```python
from build123d import *

# Parameters (mm, degrees)
F1_DEPTH = 561.975
F2_R     = 2.6162
F3_DEPTH = 25.4


with BuildPart() as f1:
    # F0 (on Right) → F1 (new body)
    with BuildSketch(Plane.YZ):
        with BuildLine():
            Line((0, -19.05), (0, -3.175))
            ThreePointArc((0, -3.175), (-0.929936, -0.929936), (-3.175, 0))
            Line((-3.175, 0), (-3.175, -25.4))
            Line((-3.175, -25.4), (22.225, -25.4))
            ThreePointArc((22.225, -25.4), (21.295064, -23.154936), (19.05, -22.225))
            Line((19.05, -22.225), (3.175, -22.225))
            ThreePointArc((3.175, -22.225), (0.929936, -21.295064), (0, -19.05))
        make_face()
    extrude(amount=-F1_DEPTH)

    # F2 (on face) → F3 (cut)
    with BuildSketch(Plane(origin=(0, 0, 0), x_dir=(-1, 0, 0), z_dir=(0, 1, 0))):
        with Locations((10.31875, -11.1125)):
            Circle(F2_R)
        with Locations((280.9875, -11.1125)):
            Circle(F2_R)
        with Locations((551.65625, -11.1125)):
            Circle(F2_R)
        with Locations((128.5875, -11.1125)):
            Circle(F2_R)
        with Locations((204.7875, -11.1125)):
            Circle(F2_R)
        with Locations((357.1875, -11.1125)):
            Circle(F2_R)
        with Locations((433.3875, -11.1125)):
            Circle(F2_R)
        with Locations((509.5875, -11.1125)):
            Circle(F2_R)
        with Locations((52.3875, -11.1125)):
            Circle(F2_R)
        with Locations((33.3375, -11.1125)):
            Circle(F2_R)
        with Locations((71.4375, -11.1125)):
            Circle(F2_R)
        with Locations((490.5375, -11.1125)):
            Circle(F2_R)
        with Locations((528.6375, -11.1125)):
            Circle(F2_R)
    extrude(amount=-F3_DEPTH, mode=Mode.SUBTRACT)


solid = f1.part
```
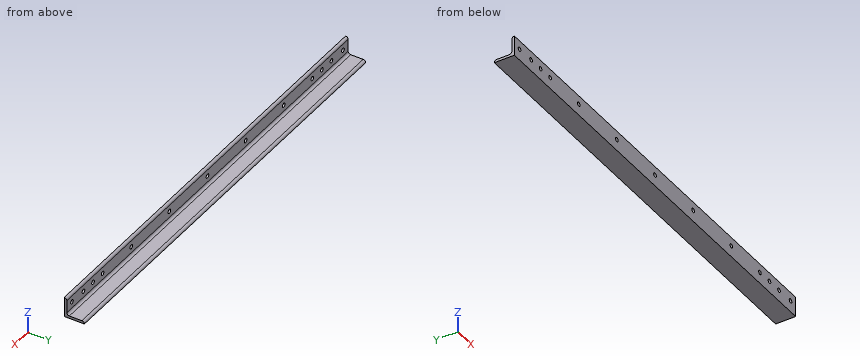
Could you check a few things on this model? Use its own coordinates, in mm. Coordinates: 2 decimals unless noted, no trailing zeros. Write each loop counter-clockwise with the first axis right and the second up, starting at its lowest first coordinate (ties: lowest second). Pieces come first, ordered by that corner, then holes. Notation, with made-up numbers: M 8,85.25 L 57,85.25 A17 ccw 57,100.25 Z; hole C 40,63.25 d4. An arc over 180 degrees is marked long. Answer as CSV lines item,"result". Start each with the question number.
1) I want a section at A-A, the plane x = -479. Please give me the cut outline in (y, z) (3 decimals).
2) For P1, Ø8, axis at y = 7, z = -11.5, coming from the +X side; P2, Ø8.5, axis at x = -10.32, z = -11.11, coming from the +Y side; P3, Ø8.5, axis at x = -33.34, z = -11.11, coming from the -Y side (3 decimals); P4, Ø3, axis at x = -364.5, y = 16, coming from the +Z side (3 decimals), each with a flat end and sliding along its axis, tell me the tip position at first contact or that it passes through.
3) Please list where these lines run through material, in increasing order: line 1 (Z direction, x = -324.5, y = 15.25) (3 decimals); line 2 (Y direction, x = -366.5, z = -16.75) (3 decimals); line 3 (Z direction, x = -401, y = 19.5). Write a range as from..to.
4) I want a section at B-B, the plane y = 15. Please give me the cut outline in (x, z) (3 decimals), and give its area (3 significant figures).
Data:
1,outline,"M -3.175,-25.4 L 22.225,-25.4 A3.175 ccw 19.05,-22.225 L 3.175,-22.225 A3.175 cw 0,-19.05 L 0,-3.175 A3.175 ccw -3.175,0 Z"
2,P1,"passes through"
2,P2,"stops at y = 0"
2,P3,"stops at y = -3.175"
2,P4,"stops at z = -22.225"
3,line 1,"z = -25.4..-22.225"
3,line 2,"y = -3.175..0"
3,line 3,"z = -25.4..-22.26"
4,outline,"M -561.975,-25.4 L 0,-25.4 L 0,-22.225 L -561.975,-22.225 Z"
4,area,"1,780 mm^2"
